Check sheet for the drawn part. Datum: minimum x, y, z corner. Units: mm. Coordinates: 2 decimals unless noted, no trailing zeros. Order: outer loops, then holes, each group sorted by start corner. A loop starts at its lowest first (then second) coordinate and runs counter-clockwise, first axis right, second up. Notation, with made-up numbers: (-2, 18.5) - (50, 18.5) arc R19 ccw to (50, 27.5) - close; hole circle Ø10 at (40, -11). An arc over 180 degrees is marked (long way). Return JSON: item names as keys, results as strings. Group by question number.
Item 1: Scan lines: probe 1 along Y at (x, z) = (5, 2.3); probe 2 along X at (y, z) = (34.5, 0.75) (3 decimals); probe 3 along Y at (x, z) = (76.5, 3.45). Record each from-to range of solid material in increasing order.
Item 2: Gauge pin test, flat end, axial feed: pin 1 (3.5 mm diameter, centred on x = 60, y = 25, fed in from -Z). Record the tip position at first contact, or that the pin passes through.
Item 3: Section check B-B on z = 2.7. Give the number of separate pieces and of enclosed holes in the cut face, then the cut area to 3 significant figures.
Item 4: Section check D-D on y = 35. Enter the section's corners in (x, z), then the cut area to 3 significant figures.
Item 5: Draft check along X on the marked faces 1 and 2. Enter one of: pulls with the +X half, pulls with the -X half, needs draft (parallel to the pull), parting line crosses it, or undercut.
Item 6: Section check C-C on x = 5. Enter the section's corners in (y, z), then the cut area to 3 significant figures.
Item 7: Section check A-A on x = 51.5. Enter the section's corners in (y, z), then the cut area to 3 significant figures.
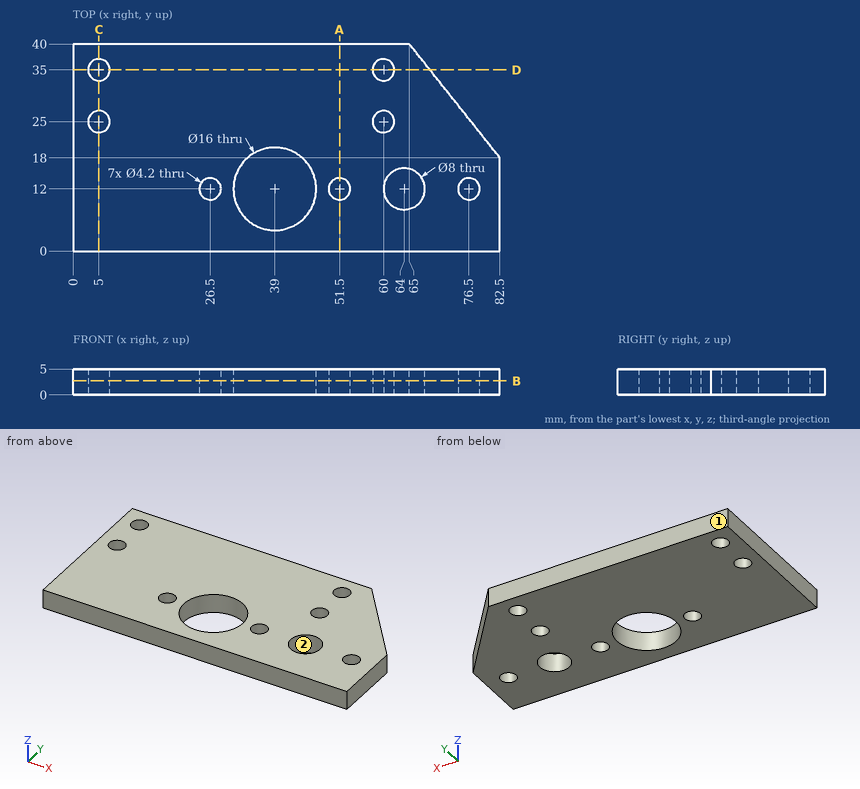
Computed:
{
 "1": {"probe 1": "y = 0 to 22.9, 27.1 to 32.9, 37.1 to 40", "probe 2": "x = 0 to 2.96, 7.04 to 57.96, 62.04 to 69.375", "probe 3": "y = 0 to 9.9, 14.1 to 25.54"},
 "2": {"pin 1": "passes through"},
 "3": {"separate pieces": "1", "enclosed holes": "9", "area": "2,760 mm²"},
 "4": {"outline": "(0, 0) - (2.9, 0) - (2.9, 5) - (0, 5) - close; (7.1, 0) - (57.9, 0) - (57.9, 5) - (7.1, 5) - close; (62.1, 0) - (68.98, 0) - (68.98, 5) - (62.1, 5) - close", "area": "303 mm²"},
 "5": {"face 1": "needs draft", "face 2": "undercut"},
 "6": {"outline": "(0, 0) - (22.9, 0) - (22.9, 5) - (0, 5) - close; (27.1, 0) - (32.9, 0) - (32.9, 5) - (27.1, 5) - close; (37.1, 0) - (40, 0) - (40, 5) - (37.1, 5) - close", "area": "158 mm²"},
 "7": {"outline": "(0, 0) - (9.9, 0) - (9.9, 5) - (0, 5) - close; (14.1, 0) - (40, 0) - (40, 5) - (14.1, 5) - close", "area": "179 mm²"}
}
